Autodesk Inventor part; units mm, degrees
ref_plane "Pracovní rovina1" through (0, 0, 91.5) normal (1, 0, 0) x (0, 0, -1)
ref_plane "Pracovní rovina2" through (-86.5, 0, 0) normal (0, 0, 1) x (1, 0, 0)
ref_plane "Pracovní rovina5" through (0, 1.75, 0) normal (0, 1, 0) x (1, 0, 0)
sketch "Náčrt1" plane through (0, 0, 0) normal (0, 1, 0) x (-1, 0, 0)
  line L0 (86.5, 91.5) -> (-86.5, 91.5)
  line L1 (-86.5, 91.5) -> (-86.5, -91.5)
  line L2 (-86.5, -91.5) -> (86.5, -91.5)
  line L3 (86.5, -91.5) -> (86.5, 91.5)
  line L4 (121.1, 0) -> (-121.1, 0)
  line L5 (0, -128.1) -> (0, 128.1)
  point P0 (0, 0)
  dimension "d0" = 183
  dimension "d1" = 173
extrude "Vysunutí1" add sketch "Náčrt1" along normal blind 3.5
sketch "Náčrt2" plane through (0, 3.5, 0) normal (0, 1, 0) x (1, 0, 0)
  circle A0 centre (-54.61, -74.259) radius 3
  line L0 (0, 128.1) -> (0, -128.1)
  line L1 (-121.1, 0) -> (121.1, 0)
  point P0 (0, 0)
  dimension "d4" = 6
  dimension "d14" = 54.61
  dimension "d15" = 74.259
extrude "Vysunutí2" add sketch "Náčrt2" along normal blind 10
ref_plane "Pracovní rovina1" through (0, 0, 91.5) normal (1, 0, 0) x (0, 0, -1)
ref_plane "Pracovní rovina2" through (-86.5, 0, 0) normal (0, 0, 1) x (1, 0, 0)
sketch "Náčrt3" plane through (-54.61, 13.5, 74.259) normal (0, 1, 0) x (1, 0, 0)
  point P0 (54.61, 74.259)
  point P1 (0, 0)
  point P2 (0, 0)
hole "Díra1" at (-54.61, 13.5, 74.259) direction (0, -1, 0) diameter 1.5 depth 8 tip angle 118
pattern_circular "Kruhové pole1" count 2 over 360 about axis through (0, -10, 0) along (0, 1, 0) of "Vysunutí2", "Díra1"
mirror "Zrcadlit1" about plane through (0, 0, 0) normal (0, 0, 1) of "Vysunutí2", "Díra1", "Kruhové pole1"
ref_plane "Pracovní rovina5" through (0, 1.75, 0) normal (0, 1, 0) x (1, 0, 0)
ref_plane "Pracovní rovina3" through (0, 0, 0) normal (0, 0, 1) x (1, 0, 0)
properties part number "Cabinet - back"
Read the model definition and answer for the solid it produces. Units are mm, in the model's axes. A direction names the side the tool comes from. Give positions to 0.01 mm unless a question says otherwise; leave off trailing zeros. Write each loop counter-clockwise with the first axis right and the second up, starting at its lowest first coordinate (ties: lowest second). Pieces come first, ordered by that corner, then holes. Notation, with made-up numbers: (74, 45.25) - (132, 45.25) arc R29 ccw to (132, 69.25) - close; hole circle Ø4 at (69, 24). An arc over 180 degrees is marked (long way). Use CSV: the item, a comma, the result in double quotes. Start each with the question number.
Item 1: A flat-ended cylindrical pin translates along its axis: P1, Ø5, axis at x = 45, y = 4, coming from the +Z side. Find the tip coordinate at first contact, or state that the pin passes through.
Item 2: Consider line 1 (Z direction, x = -54.61, y = 7.5); line 2 (Y direction, x = -72, z = -64). Determine where each line is inside the solid, lowest interval first.
Item 3: For faces 3 (the flat face through (54, 13.5, -75)), 4 (the cylindrical face through (-55.26, 8.43, 71.33)), determine the directions among +Z, -Z, +X, -X, +Y, -Y from which every point of the face is accessible in a straight line to the end or side of a thin tool.
Item 4: The mould has two halves that part along X. Classify faces 1 (the flat face through (-55.23, 13.5, -73.55)), 2 (the cylindrical face through (-55.26, 8.43, -77.188)): pulls with the +X half, pulls with the -X half, needs draft (parallel to the pull), parting line crosses it, or undercut.
Item 5: The part is cut by section A-A, the plane y = 8. Give the vertices of the cut face in (x, z).
Item 6: The part is cut by section B-B, the plane z = -29.5. Give the vertices of the cut face in (x, y), and give its area (4 significant figures).
Item 7: The part is cut by section C-C, the plane x = -28. Give the vertices of the cut face in (y, z).
Taken from the geometry:
1,P1,"z = 91.5"
2,line 1,"-77.26 to -75.01, -73.51 to -71.26, 71.26 to 73.51, 75.01 to 77.26"
2,line 2,"0 to 3.5"
3,face 3,"+Z, -Z, +X, -X, +Y"
3,face 4,"+Y"
4,face 1,"needs draft"
4,face 2,"undercut"
5,outline,"circle Ø6 at (-54.61, -74.26); circle Ø6 at (-54.61, 74.26); circle Ø6 at (54.61, -74.26); circle Ø6 at (54.61, 74.26); hole circle Ø1.5 at (-54.61, -74.26); hole circle Ø1.5 at (-54.61, 74.26); hole circle Ø1.5 at (54.61, -74.26); hole circle Ø1.5 at (54.61, 74.26)"
6,outline,"(-86.5, 0) - (86.5, 0) - (86.5, 3.5) - (-86.5, 3.5) - close"
6,area,"605.5 mm2"
7,outline,"(0, -91.5) - (3.5, -91.5) - (3.5, 91.5) - (0, 91.5) - close"
